```python
from build123d import *

# Parameters (mm, degrees)
F0_W     = 406.4
F0_H     = 76.2
F1_DEPTH = 12.7
F3_DEPTH = 25.4
F4_R     = 11.1125
F4_R_2   = 7.9375
F5_DEPTH = 25.4


with BuildPart() as f1:
    # F0 (on Top) → F1 (new body)
    with BuildSketch(Plane.XY):
        with Locations((203.2, 38.1)):
            Rectangle(F0_W, F0_H)
    extrude(amount=F1_DEPTH)

    # F2 (on face) → F3 (cut)
    with BuildSketch(Plane.XY.offset(12.7)):
        with BuildLine():
            Line((7.054568, 47.625), (0, 47.625))
            Line((0, 47.625), (0, 21.844))
            Line((0, 21.844), (7.054568, 21.844))
            ThreePointArc((7.054568, 21.844), (8.657556, 21.40963), (9.821937, 20.225373))
            ThreePointArc((9.821937, 20.225373), (15.034867, 19.509133), (14.318627, 24.722063))
            ThreePointArc((14.318627, 24.722063), (13.13437, 25.886444), (12.7, 27.489432))
            Line((12.7, 27.489432), (12.7, 41.979568))
            ThreePointArc((12.7, 41.979568), (13.13437, 43.582556), (14.318627, 44.746937))
            ThreePointArc((14.318627, 44.746937), (15.034867, 49.959867), (9.821937, 49.243627))
            ThreePointArc((9.821937, 49.243627), (8.657556, 48.05937), (7.054568, 47.625))
        make_face()
        with BuildLine():
            Line((393.7, 41.979568), (393.7, 27.489432))
            ThreePointArc((393.7, 27.489432), (393.26563, 25.886444), (392.081373, 24.722063))
            ThreePointArc((392.081373, 24.722063), (391.365133, 19.509133), (396.578063, 20.225373))
            ThreePointArc((396.578063, 20.225373), (397.742444, 21.40963), (399.345432, 21.844))
            Line((399.345432, 21.844), (406.4, 21.844))
            Line((406.4, 21.844), (406.4, 47.625))
            Line((406.4, 47.625), (399.345432, 47.625))
            ThreePointArc((399.345432, 47.625), (397.742444, 48.05937), (396.578063, 49.243627))
            ThreePointArc((396.578063, 49.243627), (391.365133, 49.959867), (392.081373, 44.746937))
            ThreePointArc((392.081373, 44.746937), (393.26563, 43.582556), (393.7, 41.979568))
        make_face()
    extrude(amount=-F3_DEPTH, mode=Mode.SUBTRACT)

    # F4 (on face) → F5 (cut)
    with BuildSketch(Plane.XY.offset(12.7)):
        with Locations((44.45, 53.975)):
            Circle(F4_R)
        with BuildLine():
            Line((55.5625, -12.145572), (55.5625, 22.225))
            ThreePointArc((55.5625, 22.225), (44.45, 33.3375), (33.3375, 22.225))
            Line((33.3375, 22.225), (33.3375, 0))
            Line((33.3375, 0), (33.3375, -12.145572))
            Line((33.3375, -12.145572), (55.5625, -12.145572))
        make_face()
        with Locations((222.25, 14.605)):
            Circle(F4_R_2)
        with Locations((247.65, 61.595)):
            Circle(F4_R_2)
        with BuildLine():
            Line((220.6625, 44.364775), (223.8375, 44.364775))
            ThreePointArc((223.8375, 44.364775), (228.327628, 46.224647), (230.1875, 50.714775))
            Line((230.1875, 50.714775), (230.1875, 63.414775))
            ThreePointArc((230.1875, 63.414775), (228.327628, 67.904903), (223.8375, 69.764775))
            Line((223.8375, 69.764775), (220.6625, 69.764775))
            ThreePointArc((220.6625, 69.764775), (216.172372, 67.904903), (214.3125, 63.414775))
            Line((214.3125, 63.414775), (214.3125, 50.714775))
            ThreePointArc((214.3125, 50.714775), (216.172372, 46.224647), (220.6625, 44.364775))
        make_face()
        with BuildLine():
            Line((246.0625, 6.4262), (249.2375, 6.4262))
            ThreePointArc((249.2375, 6.4262), (253.727628, 8.286072), (255.5875, 12.7762))
            Line((255.5875, 12.7762), (255.5875, 25.4762))
            ThreePointArc((255.5875, 25.4762), (253.727628, 29.966328), (249.2375, 31.8262))
            Line((249.2375, 31.8262), (246.0625, 31.8262))
            ThreePointArc((246.0625, 31.8262), (241.572372, 29.966328), (239.7125, 25.4762))
            Line((239.7125, 25.4762), (239.7125, 12.7762))
            ThreePointArc((239.7125, 12.7762), (241.572372, 8.286072), (246.0625, 6.4262))
        make_face()
        with BuildLine():
            Line((296.8625, 6.4262), (300.0375, 6.4262))
            ThreePointArc((300.0375, 6.4262), (304.527628, 8.286072), (306.3875, 12.7762))
            Line((306.3875, 12.7762), (306.3875, 25.4762))
            ThreePointArc((306.3875, 25.4762), (304.527628, 29.966328), (300.0375, 31.8262))
            Line((300.0375, 31.8262), (296.8625, 31.8262))
            ThreePointArc((296.8625, 31.8262), (292.372372, 29.966328), (290.5125, 25.4762))
            Line((290.5125, 25.4762), (290.5125, 12.7762))
            ThreePointArc((290.5125, 12.7762), (292.372372, 8.286072), (296.8625, 6.4262))
        make_face()
        with BuildLine():
            Line((265.1125, 63.414775), (265.1125, 50.714775))
            ThreePointArc((265.1125, 50.714775), (266.972372, 46.224647), (271.4625, 44.364775))
            Line((271.4625, 44.364775), (274.6375, 44.364775))
            ThreePointArc((274.6375, 44.364775), (279.127628, 46.224647), (280.9875, 50.714775))
            Line((280.9875, 50.714775), (280.9875, 63.414775))
            ThreePointArc((280.9875, 63.414775), (279.127628, 67.904903), (274.6375, 69.764775))
            Line((274.6375, 69.764775), (271.4625, 69.764775))
            ThreePointArc((271.4625, 69.764775), (266.972372, 67.904903), (265.1125, 63.414775))
        make_face()
        with Locations((298.45, 61.595)):
            Circle(F4_R_2)
        with Locations((273.05, 14.605)):
            Circle(F4_R_2)
        with BuildLine():
            Line((347.6625, 6.4262), (350.8375, 6.4262))
            ThreePointArc((350.8375, 6.4262), (355.327628, 8.286072), (357.1875, 12.7762))
            Line((357.1875, 12.7762), (357.1875, 25.4762))
            ThreePointArc((357.1875, 25.4762), (355.327628, 29.966328), (350.8375, 31.8262))
            Line((350.8375, 31.8262), (347.6625, 31.8262))
            ThreePointArc((347.6625, 31.8262), (343.172372, 29.966328), (341.3125, 25.4762))
            Line((341.3125, 25.4762), (341.3125, 12.7762))
            ThreePointArc((341.3125, 12.7762), (343.172372, 8.286072), (347.6625, 6.4262))
        make_face()
        with BuildLine():
            Line((315.9125, 63.414775), (315.9125, 50.714775))
            ThreePointArc((315.9125, 50.714775), (317.772372, 46.224647), (322.2625, 44.364775))
            Line((322.2625, 44.364775), (325.4375, 44.364775))
            ThreePointArc((325.4375, 44.364775), (329.927628, 46.224647), (331.7875, 50.714775))
            Line((331.7875, 50.714775), (331.7875, 63.414775))
            ThreePointArc((331.7875, 63.414775), (329.927628, 67.904903), (325.4375, 69.764775))
            Line((325.4375, 69.764775), (322.2625, 69.764775))
            ThreePointArc((322.2625, 69.764775), (317.772372, 67.904903), (315.9125, 63.414775))
        make_face()
        with Locations((349.25, 61.595)):
            Circle(F4_R_2)
        with Locations((323.85, 14.605)):
            Circle(F4_R_2)
        with BuildLine():
            Line((366.7125, 63.414775), (366.7125, 50.714775))
            ThreePointArc((366.7125, 50.714775), (368.572372, 46.224647), (373.0625, 44.364775))
            Line((373.0625, 44.364775), (376.2375, 44.364775))
            ThreePointArc((376.2375, 44.364775), (380.727628, 46.224647), (382.5875, 50.714775))
            Line((382.5875, 50.714775), (382.5875, 63.414775))
            ThreePointArc((382.5875, 63.414775), (380.727628, 67.904903), (376.2375, 69.764775))
            Line((376.2375, 69.764775), (373.0625, 69.764775))
            ThreePointArc((373.0625, 69.764775), (368.572372, 67.904903), (366.7125, 63.414775))
        make_face()
        with Locations((374.65, 14.605)):
            Circle(F4_R_2)
        with BuildLine():
            Line((90.4875, -12.145572), (90.4875, 22.225))
            ThreePointArc((90.4875, 22.225), (79.375, 33.3375), (68.2625, 22.225))
            Line((68.2625, 22.225), (68.2625, 0))
            Line((68.2625, 0), (68.2625, -12.145572))
            Line((68.2625, -12.145572), (90.4875, -12.145572))
        make_face()
        with Locations((79.375, 53.975)):
            Circle(F4_R)
        with BuildLine():
            Line((125.4125, -12.145572), (125.4125, 22.225))
            ThreePointArc((125.4125, 22.225), (114.3, 33.3375), (103.1875, 22.225))
            Line((103.1875, 22.225), (103.1875, 0))
            Line((103.1875, 0), (103.1875, -12.145572))
            Line((103.1875, -12.145572), (125.4125, -12.145572))
        make_face()
        with Locations((114.3, 53.975)):
            Circle(F4_R)
        with BuildLine():
            Line((160.3375, -12.145572), (160.3375, 22.225))
            ThreePointArc((160.3375, 22.225), (149.225, 33.3375), (138.1125, 22.225))
            Line((138.1125, 22.225), (138.1125, 0))
            Line((138.1125, 0), (138.1125, -12.145572))
            Line((138.1125, -12.145572), (160.3375, -12.145572))
        make_face()
        with Locations((149.225, 53.975)):
            Circle(F4_R)
        with BuildLine():
            Line((195.2625, -12.145572), (195.2625, 22.225))
            ThreePointArc((195.2625, 22.225), (184.15, 33.3375), (173.0375, 22.225))
            Line((173.0375, 22.225), (173.0375, 0))
            Line((173.0375, 0), (173.0375, -12.145572))
            Line((173.0375, -12.145572), (195.2625, -12.145572))
        make_face()
        with Locations((184.15, 53.975)):
            Circle(F4_R)
    extrude(amount=-F5_DEPTH, mode=Mode.SUBTRACT)


solid = f1.part
```
Here's how the part is built. I have some questions about the finished solid (model axes, mm). A direction names the side the tool comes from. Coordinates: 2 decimals unless noted, no trailing zeros. Order: outer loops, then holes, each group sorted by start corner. A loop starts at its lowest first (then second) coordinate and runs counter-clockwise, first axis right, second up. Notation, with made-up numbers: M 75,46 L 104,46 A18 cw 104,77 Z; hole C 37,-3.75 d6. An arc over 180 degrees is marked long. Answer as a JSON object with one key per item and string values. Group by question number.
(1) Suppose I cut it at A-A, the plane x = 114.3. Please give me the cut outline in (y, z), then the cut area to 3 significant figures.
(2) Suppose I cut it at B-B, the plane x = 50.5. Please give me the cut outline in (y, z), then the cut area to 3 significant figures.
(3) Suppose I cut it at C-C, the plane z = 6.75. State how many separate pieces and enclosed holes the cut face has, then the cut area to 3 significant figures.
(4) For pin 1 (5.5 mm diameter, centred on x = 4.5, z = 5, fed in from -Y), with a flat end and sliding along its axis, tell me the tip position at first contact or that it passes through.
(5) If we mould it in two halves opening along X, with no side actions, what happens to faces 3 (the face through (114.544, 33.335, 6.439)), 4 (the face through (62, 0, 6)), 5 (the face through (0, 62, 6)), 6 (the face through (184.394, 33.335, 6.439))? For each: released by +X, released by -X, zero draft, split by the parting line, or undercut.
(6) Which directions (+Z, -Z, +X, -X, +Y, -Y) give clear straight access to the entire face, cutting with the end or side of a thin tool? Please do faces 1 (the face through (33.337, 11, 6)), 2 (the face through (230.188, 57, 6)).
(7) I need wall thicknesses on probe 1 along Y at (x, z) = (349.25, 6.25); probe 2 along X at (y, z) = (42, 2); probe 3 along Y at (x, z) = (181, 5.5). Which ranges of each line are inside material? Lowest first, please.
Values found:
{
 "1": {"outline": "M 33.34,0 L 42.86,0 L 42.86,12.7 L 33.34,12.7 Z; M 65.09,0 L 76.2,0 L 76.2,12.7 L 65.09,12.7 Z", "area": "262 mm^2"},
 "2": {"outline": "M 31.55,0 L 44.65,0 L 44.65,12.7 L 31.55,12.7 Z; M 63.3,0 L 76.2,0 L 76.2,12.7 L 63.3,12.7 Z", "area": "330 mm^2"},
 "3": {"separate pieces": "1", "enclosed holes": "19", "area": "20,900 mm^2"},
 "4": {"pin 1": "stops at y = 0"},
 "5": {"face 3": "undercut", "face 4": "zero draft", "face 5": "released by -X", "face 6": "undercut"},
 "6": {"face 1": "+Z, -Z, -Y", "face 2": "+Z, -Z"},
 "7": {"probe 1": "y = 0 to 6.43, 31.83 to 53.66, 69.53 to 76.2", "probe 2": "x = 12.7 to 393.7", "probe 3": "y = 32.88 to 43.32, 64.63 to 76.2"}
}
